Could you check a few things on this model? Use its own coordinates, in mm. Give positions to 0.01 mm unless a question says otherwise; leave off trailing zeros. Loops run counter-clockwise (first coordinate to the right, second up) from the corner with the lowest first, then second, coordinate; pieces in that order, holes last. Notation, with made-up numbers: (6.25, -12) -> (57.25, -12) arc R23 cw to (57.25, -2) -> close; hole circle Ø4 at (-40, 86.5). An arc over 180 degrees is marked (long way). Write item = value, one per line. Start each with the question number.
1) I want a section at A-A (x = 200.5). List the corners of the cut face in (y, z) for me.
2) I want a section at B-B (z = -91). List the corners of the cut face in (x, y) for me.
3) I'm going to push flat-ended pins straight in: pin 1 Ø3 at (x, y) = (294, 3.5) entering from -Z; pin 2 Ø1.9 at (x, y) = (11.5, 3.5) entering from +Z; pin 3 Ø1.9 at (y, z) = (2.5, -10.5) entering from +X. Where does each tip first touch, or does it pass through?
4) I need wall thicknesses on probe 1 along X at (y, z) = (1.5, -256); probe 2 along Z at (x, y) = (80.5, 1.75). Which ranges of each line are inside material? Lowest first, please. Write a range as from..to.
from build123d import *

# Parameters (mm, degrees)
SKETCH2_W           = 38.1
SKETCH2_H           = 6.35
SKETCH2_W_2         = 25.4
SKETCH2_W_3         = 6.35
SKETCH2_H_2         = 38.1
SKETCH2_H_3         = 25.4
BOSS_EXTRUDE1_DEPTH = 6.35


with BuildPart() as part:
    # Sketch2 → Boss-Extrude1 (new body)
    with BuildSketch(Plane(origin=(0, 0, 0), x_dir=(1, 0, 0), z_dir=(0, 1, 0))):
        with Locations((57.15, -3.175)):
            Rectangle(SKETCH2_W, SKETCH2_H)
        with Locations((107.95, -3.175)):
            Rectangle(SKETCH2_W_2, SKETCH2_H)
        with Locations((184.15, -3.175)):
            Rectangle(SKETCH2_W_2, SKETCH2_H)
        with Locations((234.95, -3.175)):
            Rectangle(SKETCH2_W, SKETCH2_H)
        with Locations((295.275, 57.15)):
            Rectangle(SKETCH2_W_3, SKETCH2_H_2)
        with Locations((295.275, 107.95)):
            Rectangle(SKETCH2_W_3, SKETCH2_H_3)
        with Locations((295.275, 184.15)):
            Rectangle(SKETCH2_W_3, SKETCH2_H_3)
        with Locations((295.275, 234.95)):
            Rectangle(SKETCH2_W_3, SKETCH2_H_2)
        with Locations((234.95, 295.275)):
            Rectangle(SKETCH2_W, SKETCH2_H)
        with Locations((184.15, 295.275)):
            Rectangle(SKETCH2_W_2, SKETCH2_H)
        with Locations((107.95, 295.275)):
            Rectangle(SKETCH2_W_2, SKETCH2_H)
        with Locations((57.15, 295.275)):
            Rectangle(SKETCH2_W, SKETCH2_H)
        with Locations((-3.175, 234.95)):
            Rectangle(SKETCH2_W_3, SKETCH2_H_2)
        with Locations((-3.175, 184.15)):
            Rectangle(SKETCH2_W_3, SKETCH2_H_3)
        with Locations((-3.175, 107.95)):
            Rectangle(SKETCH2_W_3, SKETCH2_H_3)
        with Locations((-3.175, 57.15)):
            Rectangle(SKETCH2_W_3, SKETCH2_H_2)
        Polygon((0, 0), (146.05, 146.05), (0, 146.05), (0, 120.65), (0, 95.25), (0, 76.2), (0, 38.1), align=None)
        Polygon((120.65, 0), (146.05, 0), (146.05, 146.05), (0, 0), (38.1, 0), (76.2, 0), (95.25, 0), align=None)
        Polygon((146.05, 146.05), (146.05, 0), (171.45, 0), (196.85, 0), (215.9, 0), (254, 0), (292.1, 0), (292.1, 38.1), (292.1, 76.2), (292.1, 95.25), (292.1, 120.65), (292.1, 146.05), align=None)
        Polygon((292.1, 292.1), (146.05, 146.05), (292.1, 146.05), (292.1, 171.45), (292.1, 196.85), (292.1, 215.9), (292.1, 254), align=None)
        Polygon((146.05, 292.1), (146.05, 146.05), (292.1, 292.1), (254, 292.1), (215.9, 292.1), (196.85, 292.1), (171.45, 292.1), align=None)
        Polygon((0, 146.05), (146.05, 146.05), (146.05, 292.1), (120.65, 292.1), (95.25, 292.1), (76.2, 292.1), (38.1, 292.1), (0, 292.1), (0, 254), (0, 215.9), (0, 196.85), (0, 171.45), align=None)
    extrude(amount=BOSS_EXTRUDE1_DEPTH)


solid = part.part
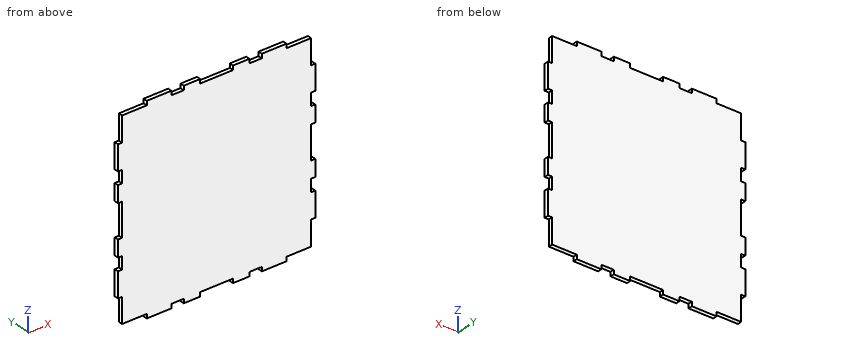
Answer list:
q1.outline = (0, -292.1) -> (6.35, -292.1) -> (6.35, 0) -> (0, 0) -> close
q2.outline = (0, 0) -> (292.1, 0) -> (292.1, 6.35) -> (0, 6.35) -> close
q3.pin_1 = -254
q3.pin_2 = 0
q3.pin_3 = 292.1
q4.probe_1 = 0..292.1
q4.probe_2 = -292.1..0
